from build123d import *

# Parameters (mm, degrees)
SKETCH1_R           = 15
BOSS_EXTRUDE1_DEPTH = 2
SKETCH2_R           = 11
SKETCH2_R_2         = 9
BOSS_EXTRUDE2_DEPTH = 35
SKETCH3_R           = 1.5
CUT_EXTRUDE1_DEPTH  = 41.926763859
FILLET1_R           = 2
FILLET2_R           = 2


with BuildPart() as part:
    # Sketch1 → Boss-Extrude1 (new body)
    with BuildSketch(Plane.XY):
        Circle(SKETCH1_R)
    extrude(amount=BOSS_EXTRUDE1_DEPTH)

    # Sketch2 → Boss-Extrude2 (add)
    with BuildSketch(Plane.XY.offset(2)):
        Circle(SKETCH2_R)
        Circle(SKETCH2_R_2, mode=Mode.SUBTRACT)
    extrude(amount=BOSS_EXTRUDE2_DEPTH)

    # Sketch3 → Cut-Extrude1 (cut, through all)
    with BuildSketch(Plane.XY.offset(2)):
        with Locations((0, 13)):
            Circle(SKETCH3_R)
        with Locations((13, 0)):
            Circle(SKETCH3_R)
        with Locations((0, -13)):
            Circle(SKETCH3_R)
        with Locations((-13, 0)):
            Circle(SKETCH3_R)
    extrude(amount=-CUT_EXTRUDE1_DEPTH, mode=Mode.SUBTRACT)

    # Fillet1
    # the kernel refuses this fillet: 2 mm, written as the material it adds along each edge
    with BuildSketch(Plane(origin=(0, 0, 2), x_dir=(1, 0, 0), z_dir=(0, -1, 0))) as fillet1_piece_1_section:
        with BuildLine():
            CenterArc((11 + FILLET1_R, FILLET1_R), FILLET1_R, 180, 90)
            Line((11, FILLET1_R), (11, 0))
            Line((11, 0), (11 + FILLET1_R, 0))
        make_face()
    fillet1_piece_1 = revolve(axis=Axis((0, 0, 2), (0, 0, 1)), mode=Mode.PRIVATE)
    fillet1_piece_1 = fillet1_piece_1 - Plane(origin=(-13, 0, 2.02819371), x_dir=(1, 0, 0), z_dir=(0, 0, 1)) * Cylinder(1.5, 52, mode=Mode.PRIVATE)
    fillet1_piece_1 = fillet1_piece_1 - Plane(origin=(0, -13, 2.02819371), x_dir=(1, 0, 0), z_dir=(0, 0, 1)) * Cylinder(1.5, 52, mode=Mode.PRIVATE)
    fillet1_piece_1 = fillet1_piece_1 - Plane(origin=(13, 0, 2.02819371), x_dir=(1, 0, 0), z_dir=(0, 0, 1)) * Cylinder(1.5, 52, mode=Mode.PRIVATE)
    fillet1_piece_1 = fillet1_piece_1 - Plane(origin=(0, 13, 2.02819371), x_dir=(1, 0, 0), z_dir=(0, 0, 1)) * Cylinder(1.5, 52, mode=Mode.PRIVATE)
    add(fillet1_piece_1)
    # the kernel refuses this fillet: 2 mm, written as the material it takes off along each edge
    with BuildSketch(Plane(origin=(0, 0, 37), x_dir=(1, 0, 0), z_dir=(0, -1, 0))) as fillet1_2_piece_1:
        with BuildLine():
            CenterArc((11 - FILLET1_R, -FILLET1_R), FILLET1_R, 0, 90)
            Line((11 - FILLET1_R, 0), (11, 0))
            Line((11, 0), (11, -FILLET1_R))
        make_face()
    revolve(axis=Axis((0, 0, 37), (0, 0, 1)), mode=Mode.SUBTRACT)

    # Fillet2
    fillet2_edges = [part.edges().sort_by_distance(p)[0] for p in [
        (-9, 0, 2),
    ]]
    fillet(fillet2_edges, radius=FILLET2_R)


solid = part.part
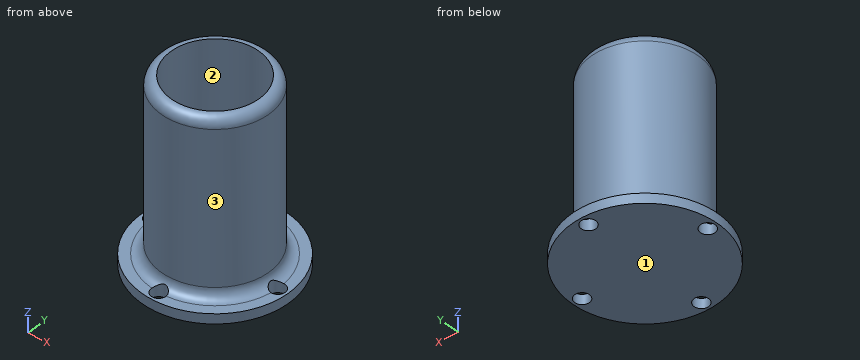
Here's how the part is built. I have some questions about the finished solid (model axes, mm). Face numbers are marked on the shaded views. Give positions to 0.01 mm unless a question says otherwise; leave off trailing zeros. Write each loop counter-clockwise with the first axis right and the second up, starting at its lowest first coordinate (ties: lowest second). Pieces come first, ordered by that corner, then holes. Notation, with made-up numbers: (75, 84) -> (90, 84) arc R20 ccw to (90, 95) -> close; hole circle Ø3 at (0.5, 50.5). An arc over 180 degrees is marked (long way). Use one line per item in the form item = value. Start each with the question number.
1. If I drill on L1, parallel to Y at x = 0, z = 1.5; L2, parallel to Y at x = 0, z = 19.5; L3, parallel to X at y = 1.5, z = 3, over which ranges is the centre line in solid material (lowest first)?
2. Will these pins go through, and if not, where does the flat tip stop? pin 1 Ø12 at (y, z) = (8, 19) entering from -X; pin 2 Ø1.5 at (y, z) = (9, 6) entering from -X; pin 3 Ø3 at (y, z) = (8, 28.5) entering from +X.
3. Imagine slicing it at C-C on z = 19. List the corners of the cut face in (x, y) for me.
4. Imagine slicing it at A-A on y = 0. List the corners of the cut face in (x, z) for me, plus the area to 3 significant figures.
5. Thinking about a two-plate mould opening in X: for the marked faces 1, 2 and 3, which applies, +X half, -X half, draft (parallel to the pull), parting line (faces both ways), or undercut?
Entries:
q1.L1 = -15 to -14.5, -11.5 to 11.5, 14.5 to 15
q1.L2 = -11 to -9, 9 to 11
q1.L3 = -11.17 to -8.6, 8.6 to 11.17
q2.pin_1 = -10.82
q2.pin_2 = -7.28
q2.pin_3 = 8.87
q3.outline = circle Ø22 at (0, 0); hole circle Ø18 at (0, 0)
q4.outline = (-15, 0) -> (-14.5, 0) -> (-14.5, 2) -> (-15, 2) -> close; (-11.5, 0) -> (11.5, 0) -> (11.5, 2.68) arc R2 cw to (11, 4) -> (11, 35) arc R2 ccw to (9, 37) -> (9, 4) arc R2 cw to (7, 2) -> (-7, 2) arc R2 cw to (-9, 4) -> (-9, 37) arc R2 ccw to (-11, 35) -> (-11, 4) arc R2 cw to (-11.5, 2.68) -> close; (14.5, 0) -> (15, 0) -> (15, 2) -> (14.5, 2) -> close
q4.area = 189 mm²
q5.face_1 = draft
q5.face_2 = undercut
q5.face_3 = parting line
